Check sheet for the modelled part. Datum: model origin and axes. Units: mm. Coordinates: 2 decimals unless noted, no trailing zeros. Loops run counter-clockwise (first coordinate to the right, second up) from the corner with the lowest first, then second, coordinate; pieces in that order, holes last. Notation, with made-up numbers: (12, 3) - (70, 3) arc R19 ccw to (70, 28) - close; hole circle Ø7 at (-17.75, -31). An arc over 180 degrees is marked (long way). Answer as a JSON object with one key per item and string values. Group by question number.
Autodesk Inventor part; units mm, degrees
ref_plane "YZ Plane" through (0, 0, 0) normal (1, 0, 0) x (0, 1, 0)
ref_plane "XZ Plane" through (0, 0, 0) normal (0, 1, 0) x (-1, 0, 0)
ref_plane "XY Plane" through (0, 0, 0) normal (0, 0, 1) x (1, 0, 0)
sketch "Sketch1" plane through (0, 0, 0) normal (0, 1, 0) x (-1, 0, 0)
  line L0 (99, -99) -> (-99, -99)
  line L1 (-99, -99) -> (-99, 99)
  line L2 (-99, 99) -> (99, 99)
  line L3 (99, 99) -> (99, -99)
  line L4 (99, -99) -> (-99, 99) construction
  line L5 (-99, -99) -> (99, 99) construction
  point P0 (0, 0)
  dimension "d0" = 198
  dimension "d1" = 198
extrude "Extrusion1" add sketch "Sketch1" along normal blind 5.88
sketch "Sketch2" plane through (0, 5.88, 0) normal (0, 1, 0) x (1, 0, 0)
  circle A0 centre (-76.175, -76.175) radius 5
  line L0 (99, 99) -> (-99, 99)
  line L1 (-99, 99) -> (-99, -99)
  line L2 (82.175, -82.175) -> (-82.175, -82.175)
  line L3 (-82.175, -82.175) -> (-82.175, 82.175)
  line L4 (-82.175, 82.175) -> (82.175, 82.175)
  line L5 (82.175, 82.175) -> (82.175, -82.175)
  line L6 (82.175, -82.175) -> (-82.175, 82.175) construction
  line L7 (-82.175, -82.175) -> (82.175, 82.175) construction
  line L8 (75, -75) -> (-75, -75)
  line L9 (-75, -75) -> (-75, 75)
  line L10 (-75, 75) -> (75, 75)
  line L11 (75, 75) -> (75, -75)
  line L12 (75, -75) -> (-75, 75) construction
  line L13 (-75, -75) -> (75, 75) construction
  circle A1 centre (-76.175, -76.175) radius 6
  circle A2 centre (-90.5875, 62.75) radius 2.5
  line L14 (0, 0) -> (-75, 0)
  circle A3 centre (-90.5875, -62.75) radius 2.5
  circle A4 centre (-62.75, -90.5875) radius 2.5
  circle A5 centre (62.75, -90.5875) radius 2.5
  circle A6 centre (90.5875, -62.75) radius 2.5
  circle A7 centre (90.5875, 62.75) radius 2.5
  circle A8 centre (62.75, 90.5875) radius 2.5
  circle A9 centre (-62.75, 90.5875) radius 2.5
  dimension "d4" = 10
  dimension "d7" = 16.825
  dimension "d8" = 16.825
  dimension "d9" = 150
  dimension "d10" = 150
  dimension "d11" = 6
  dimension "d12" = 12
  dimension "d13" = 5
  dimension "d14" = 8.4125
  dimension "d15" = 62.75
  dimension "d18" = 360
extrude "Extrusion2" [suppressed]
sketch "Sketch4" plane through (0, 0, 0) normal (0, -1, 0) x (1, 0, 0)
  line L0 (-80.5, -80.5) -> (80.5, -80.5)
  line L1 (80.5, -80.5) -> (80.5, 80.5)
  line L2 (80.5, 80.5) -> (-80.5, 80.5)
  line L3 (-80.5, 80.5) -> (-80.5, -80.5)
  line L4 (-80.5, -80.5) -> (80.5, 80.5) construction
  line L5 (80.5, -80.5) -> (-80.5, 80.5) construction
  line L6 (-100.5, -100.5) -> (100.5, -100.5)
  line L7 (100.5, -100.5) -> (100.5, 100.5)
  line L8 (100.5, 100.5) -> (-100.5, 100.5)
  line L9 (-100.5, 100.5) -> (-100.5, -100.5)
  line L10 (-100.5, -100.5) -> (100.5, 100.5) construction
  line L11 (100.5, -100.5) -> (-100.5, 100.5) construction
  circle A0 centre (-50.25, 90.5) radius 2.5
  line L12 (0, 0) -> (0, 100.5)
  circle A1 centre (50.25, 90.5) radius 2.5
  circle A2 centre (-90.5, 90.5) radius 2.5
  circle A3 centre (0, 90.5) radius 2.5
  circle A4 centre (90.5, 90.5) radius 2.5
  point P0 (0, 0)
  dimension "d20" = 201
  dimension "d21" = 201
  dimension "d22" = 20
  dimension "d23" = 20
  dimension "d24" = 5
  dimension "d25" = 50.25
  dimension "d26" = 10
  dimension "d32" = 5
  dimension "d33" = 10
  dimension "d34" = 5
  dimension "d35" = 10
extrude "Extrusion3" cut sketch "Sketch4" against normal blind 10 contours A3 L12 | L12 A3 | A0 | A1 | A2
pattern_circular "Circular Pattern1" count 4 over 360 about axis through (0, -10, 0) along (0, 1, 0) of "Extrusion3"
equation "\"d2\" = thick_acrylic"
equation "\"d4\" = stopper_diameter"
equation "\"d7\" = reservoir_overlap - 2 * sm_thickness"
equation "\"d8\" = reservoir_overlap - 2 * sm_thickness"
equation "\"d9\" = bed_x"
equation "\"d10\" = bed_y"
equation "\"d13\" = m5_diameter"
equation "\"d14\" = -sm_thickness + 0.5 * reservoir_overlap"
equation "\"d15\" = 0.25 * tray_y"
equation "\"d5\" = thick_acrylic"
equation "\"d20\" = reservoir_x"
equation "\"d21\" = reservoir_y"
equation "\"d22\" = reservoir_overlap"
equation "\"d23\" = reservoir_overlap"
equation "\"d24\" = m5_diameter"
equation "\"d25\" = 0.25 * reservoir_x"
equation "\"d26\" = 0.5 * reservoir_overlap"
equation "\"d32\" = m5_diameter"
equation "\"d33\" = 0.5 * reservoir_overlap"
equation "\"d34\" = m5_diameter"
equation "\"d35\" = 0.5 * reservoir_overlap"
equation "\"sm_thickness\" = 1.5875"
equation "\"thick_acrylic\" = 5.88"
equation "\"thin_acrylic\" = 3.15"
equation "\"clear_acrylic\" = 3.15"
equation "\"wood_thickness\" = 6.72"
equation "\"m3_diameter\" = 3"
equation "\"m4_diameter\" = 4"
equation "\"m5_diameter\" = 5"
equation "\"brass_insert_drill\" = 4"
equation "\"m5_brass_insert_drill\" = 6.7"
equation "\"m3_main_length\" = 14"
equation "\"m3_main_nut_width\" = 5.7"
equation "\"m3_main_nut_thickness\" = 2.5"
equation "\"m3_main_extra\" = 1"
equation "\"stepper_screw_space\" = 35"
equation "\"stepper_shaft_diameter\" = 5"
equation "\"stepper_body_diameter\" = 28"
equation "\"laser_body_diameter\" = 12"
equation "\"t_carrier\" = 5.88"
equation "\"t_wall\" = 5.88"
equation "\"t_window\" = 3.15"
equation "\"carrier_y\" = 251"
equation "\"carrier_z\" = 12"
equation "\"carrier_z2\" = 25"
equation "\"protection_slot\" = 36.2"
equation "\"protection_slot_offset\" = 45.25"
equation "\"window_z\" = 332.225"
equation "\"window_y\" = 93.75"
equation "\"window_slot\" = 25"
equation "\"door_sensor\" = 35"
equation "\"reservoir_x\" = 201"
equation "\"reservoir_y\" = 201"
equation "\"reservoir_overlap\" = 20"
equation "\"linear_bearing_spacing\" = 271"
equation "\"motor_spacing\" = 337"
equation "\"t_tray\" = 3.15"
equation "\"tray_border\" = 25"
equation "\"tray_x\" = 251"
equation "\"tray_y\" = 251"
equation "\"bed_x\" = 150"
equation "\"bed_y\" = 150"
equation "\"stopper_diameter\" = 10"
equation "\"brass_keep_out\" = 8"
equation "\"tape_keep_out\" = 2"
equation "\"tape_thickness\" = 2"
equation "\"t_crane\" = 6.72"
equation "\"end_stop_spacing\" = 19"
equation "\"thumb_nut_offset_y\" = 0"
equation "\"thumb_nut_diameter\" = 7"
equation "\"z_min_from_center\" = 115"
equation "\"t_frame\" = 6.72"
equation "\"frame_top_z\" = 385"
equation "\"frame_bottom_z\" = 275"
equation "\"frame_total_z\" = 661.5875"
equation "\"frame_border\" = 48.0375"
equation "\"frame_foot_z\" = 12"
equation "\"frame_tilt\" = 1deg"
equation "\"printer_z\" = 289"
equation "\"lcd_x\" = 72"
equation "\"lcd_y\" = 25"
equation "\"subframe_x\" = 66"
equation "\"subframe_y_offset\" = 27.5"
equation "\"laser_y_offset\" = 19.4"
equation "\"laser_diameter\" = 12"
equation "\"laser_z_offset\" = 55"
equation "\"laser_y\" = 15"
equation "\"laser_z\" = 75"
equation "\"t_galvo_frame\" = 6.72"
equation "\"galvo_frame_x\" = 66"
equation "\"galvo_frame_z\" = 85"
equation "\"galvo_frame_y_offset\" = 27.5"
equation "\"drawer_x\" = 257.3"
equation "\"drawer_y\" = 90.3375"
equation "\"drawer_z\" = 278.175"
equation "\"drawer_z_from_bottom\" = 25"
equation "\"crane_z2\" = 12"
equation "\"bed_z\" = 25"
equation "\"nema17_x\" = 43"
equation "\"very_thick_acrylic\" = 9.45"
equation "\"m5_press_nut_drill\" = 6.5"
equation "\"visor_x\" = 253.925"
equation "\"m3_press_nut_drill\" = 4.5"
equation "\"window_overlap\" = 48"
equation "\"m5_head\" = 10.3"
equation "\"visor_y\" = 85.6"
equation "\"door_overlap\" = 48"
equation "\"door_z\" = 332.225"
equation "\"acrylic_into_frame\" = 5"
equation "\"m3_head\" = 6"
equation "\"door_x\" = 251"
equation "\"drawer_support_from_top\" = 48"
equation "\"laser_gap\" = 1"
equation "\"frame_screw_from_center\" = 25"
equation "\"drawer_screw_from_center\" = 55"
equation "\"frame_face_y\" = 45"
equation "\"switch_spacing\" = 19"
equation "\"subframe_y\" = 55"
equation "\"al_thickness\" = 1.5875"
equation "\"rivet_diameter\" = 3.3"
equation "\"bend_factor\" = 2.26205"
equation "\"sm_bend\" = 3.591"
equation "\"al_bend\" = 3.591"
equation "\"frame_x\" = 353.375"
equation "\"carrier_y2\" = 76.825"
properties part number "tray"
1. Sectioned sample at B-B on z = 0. Record the cut outline in (x, y).
2. Sectioned sample at A-A on x = -90.5. Record the cut outline in (y, z), plus the area to 3 significant figures.
3. Release check for a two-part mould opening along Z. For faces 1 (the face through (92.98, 2.9, 90.83)), 2 (the face through (1, 5.88, 1)) record: released by +Z, released by -Z, zero draft, split by the parting line, or undercut.
4. Gauge pin test, flat ends, axial feed: pin 1 (6.5 mm diameter, centred on x = 90.5, z = -90.5, fed in from +Y); pin 2 (4 mm diameter, centred on x = -50.25, z = -90.5, fed in from +Y). Record the tip position at first contact, or that the pin passes through.
5. Material ranges on line 1 (X direction, y = 4, z = 0); line 2 (X direction, y = 2.2, z = -0.5), recorded low to high.
6. Sectioned sample at D-D on z = -90.5. Record the cut outline in (x, y), plus the area to 3 significant figures.
7. Sectioned sample at C-C on x = -50.25. Record the cut outline in (y, z), plus the area to 3 significant figures.
Answers follow:
{
 "1": {"outline": "(-99, 0) - (-93, 0) - (-93, 5.88) - (-99, 5.88) - close; (-88, 0) - (88, 0) - (88, 5.88) - (-88, 5.88) - close; (93, 0) - (99, 0) - (99, 5.88) - (93, 5.88) - close"},
 "2": {"outline": "(0, -99) - (5.88, -99) - (5.88, -93) - (0, -93) - close; (0, -88) - (5.88, -88) - (5.88, -52.75) - (0, -52.75) - close; (0, -47.75) - (5.88, -47.75) - (5.88, -2.5) - (0, -2.5) - close; (0, 2.5) - (5.88, 2.5) - (5.88, 47.75) - (0, 47.75) - close; (0, 52.75) - (5.88, 52.75) - (5.88, 88) - (0, 88) - close; (0, 93) - (5.88, 93) - (5.88, 99) - (0, 99) - close", "area": "1,020 mm^2"},
 "3": {"face 1": "undercut", "face 2": "zero draft"},
 "4": {"pin 1": "stops at y = 5.88", "pin 2": "passes through"},
 "5": {"line 1": "x = -99 to -93, -88 to 88, 93 to 99", "line 2": "x = -99 to -92.95, -88.05 to 88.05, 92.95 to 99"},
 "6": {"outline": "(-99, 0) - (-93, 0) - (-93, 5.88) - (-99, 5.88) - close; (-88, 0) - (-52.75, 0) - (-52.75, 5.88) - (-88, 5.88) - close; (-47.75, 0) - (-2.5, 0) - (-2.5, 5.88) - (-47.75, 5.88) - close; (2.5, 0) - (47.75, 0) - (47.75, 5.88) - (2.5, 5.88) - close; (52.75, 0) - (88, 0) - (88, 5.88) - (52.75, 5.88) - close; (93, 0) - (99, 0) - (99, 5.88) - (93, 5.88) - close", "area": "1,020 mm^2"},
 "7": {"outline": "(0, -99) - (5.88, -99) - (5.88, -93) - (0, -93) - close; (0, -88) - (5.88, -88) - (5.88, 88) - (0, 88) - close; (0, 93) - (5.88, 93) - (5.88, 99) - (0, 99) - close", "area": "1,110 mm^2"}
}
